from build123d import *

# Parameters (mm, degrees)
F0_R      = 57.15
F1_DEPTH  = 50.8
F3_DEPTH  = 19.558
F3_TAPER  = -20
F4_R      = 6.2936764169
F4_R_2    = 4.5582731786
F4_R_3    = 3.0215351301
F4_R_4    = 4.2985160405
F4_R_5    = 2.3322780101
F4_R_6    = 3.1916024355
F4_R_7    = 2.0879014362
F4_R_8    = 5.5078897411
F4_R_9    = 1.5847885442
F5_DEPTH  = 16.51
F6_R      = 3.5004361301
F7_DEPTH  = 8.89
F8_R      = 5.08
F9_R      = 5.08
F10_R     = 5.08
F11_R     = 9.1016628177
F12_DEPTH = 31.2430001


with BuildPart() as f1:
    # F0 (on Front) → F1 (new body)
    with BuildSketch(Plane.XZ):
        Circle(F0_R)
    extrude(amount=F1_DEPTH)

    # F2 (on face) → F3 (cut)
    with BuildSketch(Plane.XZ.offset(50.8)):
        with BuildLine():
            Line((56.6691125389, 7.398255474), (-56.6691125389, 7.398255474))
            ThreePointArc((-56.6691125389, 7.398255474), (-57.103483703, -2.3053522456), (-55.8883030293, -11.9423651134))
            Line((-55.8883030293, -11.9423651134), (55.8883030293, -11.9423651134))
            ThreePointArc((55.8883030293, -11.9423651134), (56.8337004696, -6.0044142876), (57.15, 0))
            ThreePointArc((57.15, 0), (57.0296514175, 3.7069339355), (56.6691125389, 7.398255474))
        make_face()
    extrude(amount=-F3_DEPTH, taper=F3_TAPER, mode=Mode.SUBTRACT)

    # F4 (on face) → F5 (cut)
    with BuildSketch(Plane.XZ.offset(50.8)):
        with Locations((-33.159788698, 30.5929593742)):
            Circle(F4_R)
        with Locations((-14.6182132885, 30.5929593742)):
            Circle(F4_R_2)
        with Locations((27.5545194745, -26.9502550364)):
            Circle(F4_R_3)
        with Locations((5.0058867782, -36.4746116102)):
            Circle(F4_R_4)
        with Locations((-27.5286901742, -20.31073533)):
            Circle(F4_R_5)
        with Locations((9.0075330809, 16.3046922535)):
            Circle(F4_R_6)
        with Locations((8.5346112028, 40.4698885977)):
            Circle(F4_R_7)
        with Locations((28.0849561095, 24.853952229)):
            Circle(F4_R_8)
        Polygon((-9.5280949026, -41.6518002748), (-21.0372693837, -29.4488035142), (-54.37650159, -29.4488035142), (-54.37650159, -41.6518002748), align=None)
        with Locations((-12.0945619419, 44.4322191179)):
            Circle(F4_R_9)
    extrude(amount=-F5_DEPTH, mode=Mode.SUBTRACT)

    # F6 (on face) → F7 (join)
    with BuildSketch(Plane.XZ.offset(34.29)):
        with Locations((-29.2805414647, -34.9123850465)):
            Circle(F6_R)
    extrude(amount=F7_DEPTH)

    # F8
    f8_edges = [f1.edges().sort_by_distance(p)[0] for p in [
        (17.054702, -50.8, -54.545941),
    ]]
    fillet(f8_edges, radius=F8_R)

    # F9
    f9_edges = [f1.edges().sort_by_distance(p)[0] for p in [
        (0, -50.8, 57.15),
    ]]
    fillet(f9_edges, radius=F9_R)

    # F10
    f10_edges = [f1.edges().sort_by_distance(p)[0] for p in [
        (-53.158996, -50.8, -20.981984),
    ]]
    fillet(f10_edges, radius=F10_R)

    # F11 (on face) → F12 (cut, through all)
    with BuildSketch(Plane.XZ.offset(31.242)):
        Circle(F11_R)
    extrude(amount=-F12_DEPTH, mode=Mode.SUBTRACT)


solid = f1.part
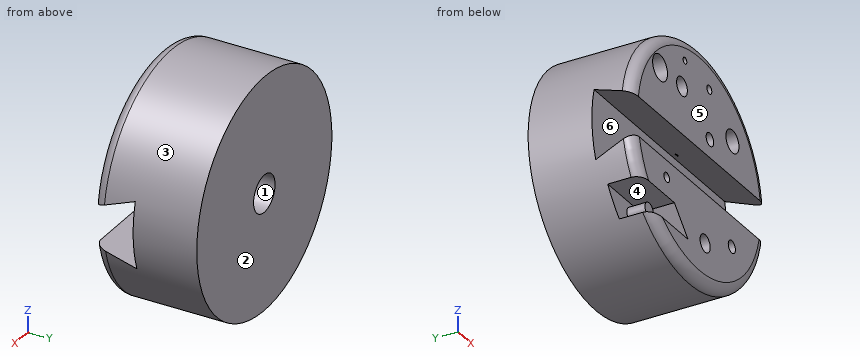
Design review of the part built by this model. Coordinates are the model's own, in mm. Face numbers are marked on the shaded views. A direction names the side the tool comes from. Coordinates: 2 decimals unless noted, no trailing zeros. Order: outer loops, then holes, each group sorted by start corner. A loop starts at its lowest first (then second) coordinate and runs counter-clockwise, first axis right, second up.
Item 1: For line 1 (X direction, y = -36, z = 28.5); line 2 (Y direction, x = -38, z = 31.5); line 3 (Z direction, x = 0, y = -16), list the stretches that pass through material, from the lowest coordinate up.
Item 2: For the marked faces 4, 5 and 6, list the 3-axis set-ups (+Z, -Z, +X, -X, +Y, -Y) from which the entire face can be reached by the end or side of a thin tool; tool diameter is ignored.
Item 3: Take a section at B-B, the plane y = -18. Write out the cut boundary in (x, z).
Item 4: The part is to be moulded in two halves that separate along Z. For the marked faces 1, 2 and 3, say which applies: pulls with the +Z half, pulls with the -Z half, needs draft (parallel to the pull), parting line crosses it, or undercut.
Item 5: Take a section at A-A, the plane z = 0. Write out the cut boundary in (x, y), then the cut area to 3 significant figures.
Item 6: For pin 1 Ø8 at (y, z) = (-12, -44.5) entering from -X; pin 2 Ø1.5 at (x, y) = (-6, -42.5) entering from -Z; pin 3 Ø5 at (x, z) = (27.55, -26.95) entering from -Y, all flat-tipped, find the tip position at first contact; note any pin that passes through.
The answers:
1. line 1: x = -49.54 to -39.1, -27.22 to -18.67, -10.57 to 23.96, 32.21 to 49.54
1. line 2: y = -34.29 to 0
1. line 3: z = -57.15 to -9.1, 9.1 to 57.15
2. face 4: -X, -Y
2. face 5: +Z, -Z, +X, -X, -Y
2. face 6: +X, -X
3. outline: circle Ø114.3 at (0, 0); hole circle Ø18.2 at (0, 0)
4. face 1: undercut
4. face 2: needs draft
4. face 3: parting line crosses it
5. outline: (-57.15, -31.24) - (-9.1, -31.24) - (-9.1, 0) - (-57.15, 0) - close; (9.1, -31.24) - (57.15, -31.24) - (57.15, 0) - (9.1, 0) - close
5. area: 3,000 mm2
6. pin 1: stops at x = -40.32
6. pin 2: stops at z = -56.91
6. pin 3: stops at y = -34.29
